Study the drawing (mm; zero at the part's minimum x, y, z) and answer. A direction names the side the tool comes from. Give positions to 0.01 mm unless a question says otherwise; leave off trailing zeros. Write each loop counter-clockwise with the first axis right and the second up, starting at its lowest first coordinate (ties: lowest second). Pieces come first, ordered by that corner, then holes. Notation, with made-up numbers: (82, -11) - (112, -11) arc R19 cw to (112, 18) - close; hole circle Ø11 at (30, -20). An arc over 180 degrees is marked (long way). Answer in a Markdown table with one row per item. Add a question column.
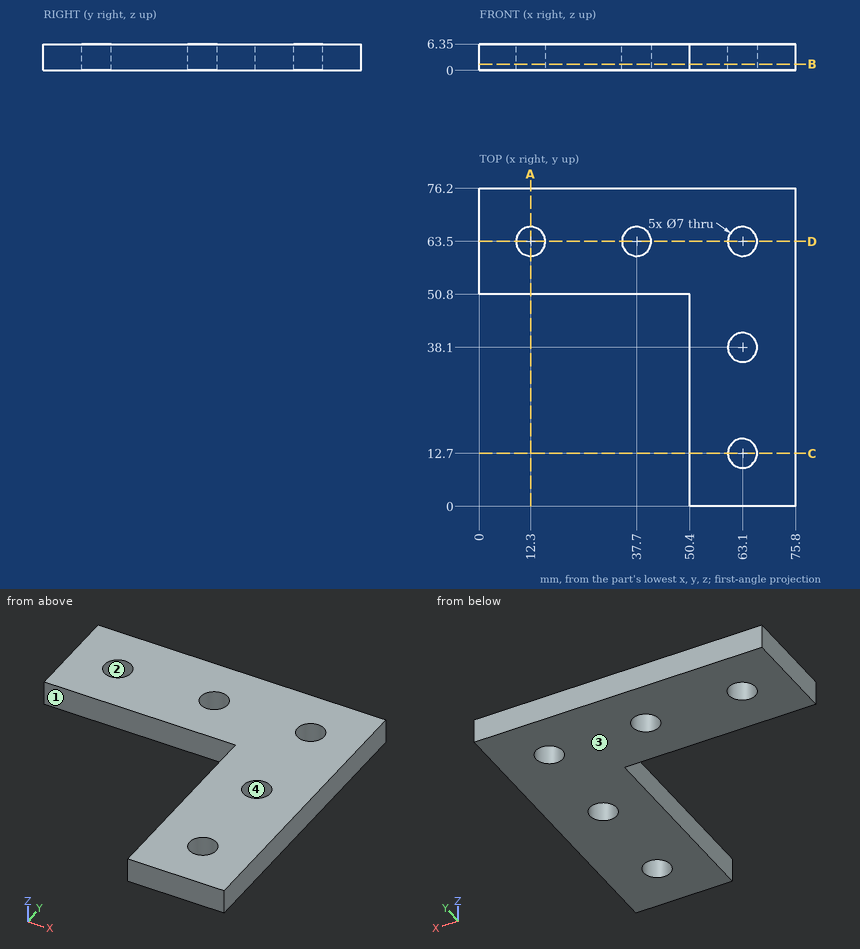
1. Given pin 1 Ø3 at (y, z) = (33.5, 5.5) entering from -X, flat-ended and moving along its own axis, determine where the tip first touches the part or whether it passes through.
2. The mould has two halves that part along X. Classify the marked faces 3 and 4: +X half, -X half, draft (parallel to the pull), parting line (faces both ways), or undercut.
3. A tool of negligible diameter and unlimited length cuts with its end or side. For the marked faces 1 and 2, from which of +Z, -Z, +X, -X, +Y, -Y can it reach the whole face along a straight path? Write none if from no direction.
4. Section C-C (y = 12.7) is taken. Give the vertices of the cut face in (x, z), and give its area (3 significant figures).
5. Section A-A (x = 12.3) is taken. Give the vertices of the cut face in (y, z), and give its area (3 significant figures).
6. Section D-D (y = 63.5) is taken. Give the vertices of the cut face in (x, z), and give its area (3 significant figures).
7. Straight lines are drawn through the part: L1, parallel to X at y = 64.5, z = 0.75; L2, parallel to Y at x = 12.3, z = 3; L3, parallel to Y at x = 61.5, z = 2. For each, find the intervals that lie inside material, in ascending order. Write a range as [from, to].
8. Section B-B (z = 1.5) is taken. Give the vertices of the cut face in (x, y).
Geometry check:
| question | item | result |
|---|---|---|
| 1 | pin 1 | x = 50.4 |
| 2 | face 3 | draft |
| 2 | face 4 | undercut |
| 3 | face 1 | +Z, -Z, -X, -Y |
| 3 | face 2 | +Z, -Z |
| 4 | outline | (50.4, 0) - (59.6, 0) - (59.6, 6.35) - (50.4, 6.35) - close; (66.6, 0) - (75.8, 0) - (75.8, 6.35) - (66.6, 6.35) - close |
| 4 | area | 117 mm² |
| 5 | outline | (50.8, 0) - (60, 0) - (60, 6.35) - (50.8, 6.35) - close; (67, 0) - (76.2, 0) - (76.2, 6.35) - (67, 6.35) - close |
| 5 | area | 117 mm² |
| 6 | outline | (0, 0) - (8.8, 0) - (8.8, 6.35) - (0, 6.35) - close; (15.8, 0) - (34.2, 0) - (34.2, 6.35) - (15.8, 6.35) - close; (41.2, 0) - (59.6, 0) - (59.6, 6.35) - (41.2, 6.35) - close; (66.6, 0) - (75.8, 0) - (75.8, 6.35) - (66.6, 6.35) - close |
| 6 | area | 348 mm² |
| 7 | L1 | [0, 8.95], [15.65, 34.35], [41.05, 59.75], [66.45, 75.8] |
| 7 | L2 | [50.8, 60], [67, 76.2] |
| 7 | L3 | [0, 9.59], [15.81, 34.99], [41.21, 60.39], [66.61, 76.2] |
| 8 | outline | (0, 50.8) - (50.4, 50.8) - (50.4, 0) - (75.8, 0) - (75.8, 76.2) - (0, 76.2) - close; hole circle Ø7 at (12.3, 63.5); hole circle Ø7 at (37.7, 63.5); hole circle Ø7 at (63.1, 12.7); hole circle Ø7 at (63.1, 38.1); hole circle Ø7 at (63.1, 63.5) |
